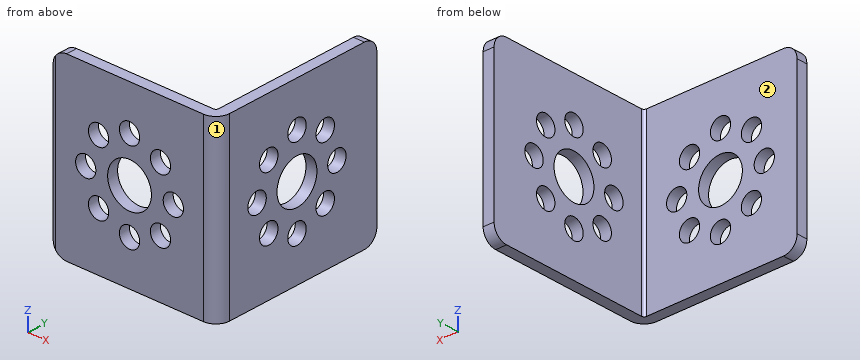
```python
from build123d import *

# Parameters (mm, degrees)
EXTRUDE1_DEPTH     = 16
FILLET1_R          = 2.5
SKETCH2_R          = 4
CUT_EXTRUDE1_DEPTH = 40.191835885
SKETCH3_R          = 4
CUT_EXTRUDE3_DEPTH = 49
SKETCH3_3_R        = 1.85
CUT_EXTRUDE4_DEPTH = 49
SKETCH2_4_R        = 1.85
CUT_EXTRUDE2_DEPTH = 40.191835885
CIRPATTERN1_COUNT  = 8
CIRPATTERN3_COUNT  = 8
CUT_EXTRUDE5_DEPTH = 49
CUT_EXTRUDE7_DEPTH = 49
FILLET2_R          = 2.5


with BuildPart() as part:
    # Sketch1 → Extrude1 (new, symmetric)
    with BuildSketch(Plane.XY):
        with BuildLine():
            Line((-13.5, 0), (13.5, 0))
            ThreePointArc((13.5, 0), (15.267766953, 0.732233047), (16, 2.5))
            Line((16, 2.5), (16, 32))
            Line((16, 32), (14, 32))
            Line((14, 32), (14, 2.5))
            ThreePointArc((14, 2.5), (13.853553391, 2.146446609), (13.5, 2))
            Line((13.5, 2), (-13.5, 2))
            ThreePointArc((-13.5, 2), (-13.853553391, 2.146446609), (-14, 2.5))
            Line((-14, 2.5), (-14, 32))
            Line((-14, 32), (-16, 32))
            Line((-16, 32), (-16, 2.5))
            ThreePointArc((-16, 2.5), (-15.267766953, 0.732233047), (-13.5, 0))
        make_face()
    extrude(amount=EXTRUDE1_DEPTH, both=True)

    # Fillet1
    fillet1_edges = [part.edges().sort_by_distance(p)[0] for p in [
        (-15, 32, -16),
        (-15, 32, 16),
        (15, 32, -16),
        (15, 32, 16),
    ]]
    fillet(fillet1_edges, radius=FILLET1_R)

    # Sketch2 → Cut-Extrude1 (cut, through all)
    with BuildSketch(Plane.XZ):
        Circle(SKETCH2_R)
    extrude(amount=-CUT_EXTRUDE1_DEPTH, mode=Mode.SUBTRACT)

    # Sketch3 → Cut-Extrude3 (cut, through all)
    with BuildSketch(Plane.ZY.offset(16)):
        with Locations(Location((0, 16, 0), (0, 0, 270))):
            Circle(SKETCH3_R)
    extrude(amount=-CUT_EXTRUDE3_DEPTH, mode=Mode.SUBTRACT)

    # Sketch3<3> → Cut-Extrude4 (cut, through all)
    with BuildSketch(Plane.ZY.offset(16)):
        with Locations(Location((0, 8, 0), (0, 0, 270))):
            Circle(SKETCH3_3_R)
    cut_extrude4 = extrude(amount=-CUT_EXTRUDE4_DEPTH, mode=Mode.SUBTRACT)

    # Sketch2<4> → Cut-Extrude2 (cut, through all)
    with BuildSketch(Plane.XZ):
        with Locations((8, 0)):
            Circle(SKETCH2_4_R)
    cut_extrude2 = extrude(amount=-CUT_EXTRUDE2_DEPTH, mode=Mode.SUBTRACT)

    # CirPattern1: Cut-Extrude2 ×8 about axis
    cirpattern1_axis = Axis((0, 0, 0), (0, 1, 0))
    for i in range(1, CIRPATTERN1_COUNT):
        add(cut_extrude2.rotate(cirpattern1_axis, i * 360 / CIRPATTERN1_COUNT), mode=Mode.SUBTRACT)

    # CirPattern3: Cut-Extrude4 ×8 about axis
    cirpattern3_axis = Axis((0, 16, 0), (1, 0, 0))
    for i in range(1, CIRPATTERN3_COUNT):
        add(cut_extrude4.rotate(cirpattern3_axis, i * 360 / CIRPATTERN3_COUNT), mode=Mode.SUBTRACT)

    # Sketch4 → Cut-Extrude5 (cut, through all)
    with BuildSketch(Plane(origin=(0, 0, -16), x_dir=(-1, 0, 0), z_dir=(0, 0, -1))):
        with BuildLine():
            Line((14, 29.5), (14, 2.5))
            Line((14, 2.5), (14, 0.050510257))
            ThreePointArc((14, 0.050510257), (15.436491673, 0.91886117), (16, 2.5))
            Line((16, 2.5), (16, 29.5))
            Line((16, 29.5), (14, 29.5))
        make_face()
        with BuildLine():
            ThreePointArc((16, 2.5), (15.436491673, 0.91886117), (14, 0.050510257))
            Line((14, 0.050510257), (14, -1.144356578))
            Line((14, -1.144356578), (16.915765157, -1.144356578))
            Line((16.915765157, -1.144356578), (16.915765157, 33.185918655))
            Line((16.915765157, 33.185918655), (14, 33.185918655))
            Line((14, 33.185918655), (14, 29.5))
            Line((14, 29.5), (16, 29.5))
            Line((16, 29.5), (16, 2.5))
        make_face()
    extrude(amount=-CUT_EXTRUDE5_DEPTH, mode=Mode.SUBTRACT)

    # Sketch5 → Cut-Extrude7 (cut, through all)
    with BuildSketch(Plane(origin=(0, 0, -16), x_dir=(-1, 0, 0), z_dir=(0, 0, -1))):
        Polygon((13.5, 2), (15.292334009, 2), (14.396167004, 3.92414695), align=None)
    extrude(amount=-CUT_EXTRUDE7_DEPTH, mode=Mode.SUBTRACT)

    # Fillet2
    fillet2_edges = [part.edges().sort_by_distance(p)[0] for p in [
        (-14, 1.025255129, 16),
        (-14, 1.025255129, -16),
    ]]
    fillet(fillet2_edges, radius=FILLET2_R)


solid = part.part
```
CAD build for the part. Positions are in the model's coordinates, mm. Face numbers are marked on the shaded views. A direction names the side the tool comes from. Round coordinates to 2 decimals unless told otherwise and drop trailing zeros. Loops run counter-clockwise (first coordinate to the right, second up) from the corner with the lowest first, then second, coordinate; pieces in that order, holes last. Notation, with made-up numbers: M 16,-36.75 L 31,-36.75 A20 ccw 31,-7.75 Z; hole C -19.5,57.5 d1. An arc over 180 degrees is marked long. Use a Markdown table: item, result. Add a question column.
(1) Drill centre lines: line 1 (X direction, y = 30, z = -9); line 2 (Y direction, x = -0.5, z = 13.5). Where is each one in solid material? Low to high.
(2) Cut at C-C (y = 16). Give the cut face in (x, z), and give its area (3 significant figures).
(3) Cut at D-D (x = 0). Give the cut face in (y, z).
(4) Flat gauge pins, fed straight in: pin 1 (5 mm diameter, centred on x = 0, z = -8, fed in from +Y); pin 2 (6.5 mm diameter, centred on x = 0, z = 0, fed in from +Y); pin 3 (15 mm diameter, centred on y = 14, z = -1.5, fed in from -X). Where does each tip first touch, or does it go through?
(5) Which spindle directions (+Z, -Z, +X, -X, +Y, -Y) get a long thin tool onto all of the face, cutting with end or side? Do the marked faces 1 and 2. Say none if no direction does.
(6) Cut at A-A (z = -8). Give the cut face in (x, y), and give its area (3 significant figures).
(7) Cut at B-B (x = 8). Give the cut face in (y, z), and give its area (3 significant figures).
Geometry says:
| question | item | result |
|---|---|---|
| 1 | line 1 | x = 14 to 16 |
| 1 | line 2 | y = 0 to 2 |
| 2 | outline | M 14,-16 L 16,-16 L 16,-9.85 L 14,-9.85 Z; M 14,-6.15 L 16,-6.15 L 16,-4 L 14,-4 Z; M 14,4 L 16,4 L 16,6.15 L 14,6.15 Z; M 14,9.85 L 16,9.85 L 16,16 L 14,16 Z |
| 2 | area | 33.2 mm² |
| 3 | outline | M 0,-16 L 2,-16 L 2,-9.85 L 0,-9.85 Z; M 0,-6.15 L 2,-6.15 L 2,-4 L 0,-4 Z; M 0,4 L 2,4 L 2,6.15 L 0,6.15 Z; M 0,9.85 L 2,9.85 L 2,16 L 0,16 Z |
| 4 | pin 1 | stops at y = 2 |
| 4 | pin 2 | passes through |
| 4 | pin 3 | stops at x = 14 |
| 5 | face 1 | +Z, -Z, +X, -Y |
| 5 | face 2 | +Z, -Z, -X, +Y |
| 6 | outline | M -14,0.05 A2.5 ccw -13.5,0 L -1.85,0 L -1.85,2 L -14,2 Z; M 1.85,0 L 13.5,0 A2.5 ccw 16,2.5 L 16,14.15 L 14,14.15 L 14,2.5 A0.5 cw 13.5,2 L 1.85,2 Z; M 14,17.85 L 16,17.85 L 16,32 L 14,32 Z |
| 6 | area | 104 mm² |
| 7 | outline | M 0,-16 L 2,-16 L 2,-1.85 L 0,-1.85 Z; M 0,1.85 L 2,1.85 L 2,16 L 0,16 Z |
| 7 | area | 56.6 mm² |
